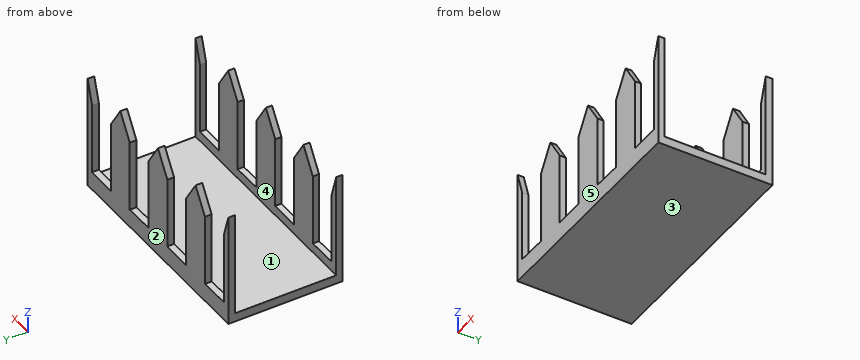
from build123d import *

# Parameters (mm, degrees)
F1_DEPTH = 76.2
F2_W     = 67.586093
F2_H     = 79.264563
F3_DEPTH = 177.8


with BuildPart() as f1:
    # F0 (on Front) → F1 (new body)
    with BuildSketch(Plane.XZ):
        Polygon((0, 76.2), (0, 0), (76.2, 0), (76.2, 76.2), (71.288093, 60.266774), (71.288093, 48.327021), (71.288093, 12.505721), (50.920066, 12.174042), (50.920066, 48.327021), (50.920066, 60.266774), (40.736053, 76.2), (30.55204, 60.266774), (30.55204, 48.327021), (30.55204, 12.174042), (10.184013, 12.505721), (10.184013, 48.327021), (10.184013, 60.266774), align=None)
        Polygon((-76.2, 0), (0, 0), (0, 76.2), (-10.184013, 60.266774), (-10.184013, 48.327021), (-10.184013, 12.505721), (-30.55204, 12.174042), (-30.55204, 48.327021), (-30.55204, 60.266774), (-40.736053, 76.2), (-50.920066, 60.266774), (-50.920066, 48.327021), (-50.920066, 12.174042), (-71.288093, 12.505721), (-71.288093, 48.327021), (-71.288093, 60.266774), (-76.2, 76.2), align=None)
    extrude(amount=F1_DEPTH)

    # F2 (on face) → F3 (cut)
    with BuildSketch(Plane.YZ.offset(76.2)):
        with Locations((-38.265653, 45.471521)):
            Rectangle(F2_W, F2_H)
    extrude(amount=-F3_DEPTH, mode=Mode.SUBTRACT)


solid = f1.part
Part model, mm, in its own coordinate system. Face numbers are marked on the shaded views. A direction names the side the tool comes from. Give positions to 0.01 mm unless a question says otherwise; leave off trailing zeros. Loops run counter-clockwise (first coordinate to the right, second up) from the corner with the lowest first, then second, coordinate; pieces in that order, holes last.
(1) Drill centre lines: line 1 along Y through (x, z) = (33, 29.5); line 2 along Z through (x, y) = (-36, -25). Where is each one in solid material? Low to high.
Return value:
line 1: y = -76.2 to -72.06, -4.47 to 0
line 2: z = 0 to 5.84
(2) Band-saw the part on D-D (x = -17). Write the cut outline in (y, z).
Return value:
outline: (-76.2, 0) - (0, 0) - (0, 12.39) - (-4.47, 12.39) - (-4.47, 5.84) - (-72.06, 5.84) - (-72.06, 12.39) - (-76.2, 12.39) - close
(3) Pull direction Y, two halves, no side cores. Call the marked faces 1, 2 and 3: pulls with the +Y half, pulls with the -Y half, needs draft (parallel to the pull), parting line crosses it, or undercut.
Return value:
face 1: undercut
face 2: pulls with the +Y half
face 3: needs draft
(4) Band-saw the part on B-B (z = 32). Count the separate pieces of the cut face and the enclosed holes in it, and give its area (3 significant figures).
Return value:
separate pieces: 10
enclosed holes: 0
area: 611 mm2
(5) Band-saw the part on A-A (x = 61). Write the cut outline in (y, z), and give its area (3 significant figures).
Return value:
outline: (-76.2, 0) - (0, 0) - (0, 12.34) - (-4.47, 12.34) - (-4.47, 5.84) - (-72.06, 5.84) - (-72.06, 12.34) - (-76.2, 12.34) - close
area: 501 mm2
(6) 3-axis set-ups, long thin cutter, end or side, ignore diameter. For the marked faces 4 and 5: which of +Z, -Z, +X, -X, +Y, -Y reach the whole face in a straight line?
Return value:
face 4: +Z, +X, -X
face 5: +Z, -Z, +X, -X, -Y
(7) Band-saw the part on C-C (y = -25). Write the cut outline in (x, z), and give its area (3 significant figures).
Return value:
outline: (-76.2, 0) - (76.2, 0) - (76.2, 5.84) - (-76.2, 5.84) - close
area: 890 mm2
(8) Pin check, flat tip, straight feed: pin 1 (3 mm diameter, centred on x = -26.5, y = -61.5, fed in from +Z). Stop position of the tip, or through.
Return value:
pin 1: stops at z = 5.84
